from build123d import *

# Parameters (mm, degrees)
BOSS_EXTRUDE1_DEPTH          = 75
SKETCH2_R                    = 2
CUT_EXTRUDE1_DEPTH           = 15
SKETCH4_R                    = 2
CUT_EXTRUDE2_DEPTH           = 12
SKETCH3_R                    = 2.3876
CUT_EXTRUDE3_DEPTH           = 6.35
CUT_EXTRUDE3_DRAFT           = -8
CUT_EXTRUDE3_PROFILE_2_DEPTH = 6.35
CUT_EXTRUDE3_PROFILE_2_DRAFT = -8
CUT_EXTRUDE4_START           = -3
CUT_EXTRUDE4_DEPTH           = 3
CUT_EXTRUDE5_START           = -3
CUT_EXTRUDE5_DEPTH           = 3
CUT_EXTRUDE6_START           = -3
CUT_EXTRUDE6_DEPTH           = 3
CUT_EXTRUDE7_START           = -3
CUT_EXTRUDE7_DEPTH           = 3
SKETCH9_R                    = 1.4951657
CUT_EXTRUDE8_DEPTH           = 5
MIRROR2_COPY_1_SKETCH_R      = 2.3876
MIRROR2_COPY_1_DEPTH         = 6.35
MIRROR2_COPY_1_DRAFT         = -8
MIRROR2_COPY_2_SKETCH_R      = 2.3876
MIRROR2_COPY_2_DEPTH         = 6.35
MIRROR2_COPY_2_DRAFT         = -8
MIRROR2_COPY_3_SKETCH_R      = 2.3876
MIRROR2_COPY_3_DEPTH         = 6.35
MIRROR2_COPY_3_DRAFT         = -8
FILLET2_START                = 9
FILLET2_DEPTH                = 4.666666667
FILLET2_START_2              = 4
FILLET2_2_DEPTH              = 39
FILLET3_R                    = 2
SKETCH10_W                   = 1.7
SKETCH10_H                   = 63
CUT_EXTRUDE9_DEPTH           = 5
FILLET4_R                    = 1
SKETCH11_W                   = 10.2
SKETCH11_H                   = 17.7
CUT_EXTRUDE10_DEPTH          = 15
SKETCH12_R                   = 1.397
CUT_EXTRUDE11_DEPTH          = 10
FILLET5_R                    = 1
CUT_EXTRUDE12_START          = -5
CUT_EXTRUDE12_DEPTH          = 3


with BuildPart() as part:
    # Sketch1 → Boss-Extrude1 (new body)
    with BuildSketch(Plane(origin=(0, 0, 0), x_dir=(1, 0, 0), z_dir=(0, 1, 0))):
        with BuildLine():
            Line((-6.825, -6.666666667), (-6.825, -26.666666667))
            Line((-6.825, -26.666666667), (8.175, -26.666666667))
            Line((8.175, -26.666666667), (8.175, -13.175))
            Line((8.175, -13.175), (60, -13.175))
            Line((60, -13.175), (60, -1.175))
            Line((60, -1.175), (25, -1.175))
            Line((25, -1.175), (25, 2))
            ThreePointArc((25, 2), (14.923352523, 3.572976633), (5.805515239, 8.142235123))
            ThreePointArc((5.805515239, 8.142235123), (3.047757271, 9.524241472), (0, 10))
            ThreePointArc((0, 10), (-7.071067812, 7.071067812), (-10, 0))
            Line((-10, 0), (-10, -6.666666667))
            Line((-10, -6.666666667), (-6.825, -6.666666667))
        make_face()
    extrude(amount=BOSS_EXTRUDE1_DEPTH)

    # Sketch2 → Cut-Extrude1 (cut)
    with BuildSketch(Plane.ZY.offset(6.825)):
        with Locations((15.666666667, 65)):
            Circle(SKETCH2_R)
    cut_extrude1 = extrude(amount=-CUT_EXTRUDE1_DEPTH, mode=Mode.SUBTRACT)

    # Sketch4 → Cut-Extrude2 (cut)
    with BuildSketch(Plane(origin=(0, 0, 1.175), x_dir=(-1, 0, 0), z_dir=(0, 0, -1))):
        with Locations((-45, 65)):
            Circle(SKETCH4_R)
    cut_extrude2 = extrude(amount=-CUT_EXTRUDE2_DEPTH, mode=Mode.SUBTRACT)


with BuildPart() as cut_extrude3_tool:
    # Sketch3 → Cut-Extrude3 (with draft: the straight prism first)
    with BuildSketch(Plane(origin=(0, 75, 0), x_dir=(1, 0, 0), z_dir=(0, 1, 0))):
        with Locations((1, -1)):
            Circle(SKETCH3_R)
    extrude(amount=-CUT_EXTRUDE3_DEPTH)
    # Cut-Extrude3: the draft: its side faces are tilted about the plane it starts from
    cut_extrude3_sides = [cut_extrude3_tool.faces().sort_by_distance(p)[0] for p in [
        (-1.3876, 71.825, 1),
    ]]
    draft(cut_extrude3_sides, Plane(origin=(0, 75, 0), x_dir=(1, 0, 0), z_dir=(0, 1, 0)), CUT_EXTRUDE3_DRAFT)


with BuildPart() as part_1:
    add(part.part)

    # Cut-Extrude3: cut by cut_extrude3_tool
    add(cut_extrude3_tool.part, mode=Mode.SUBTRACT)


with BuildPart() as cut_extrude3_profile_2_tool:
    # Sketch3 → Cut-Extrude3 profile 2 (with draft: the straight prism first)
    with BuildSketch(Plane(origin=(0, 75, 0), x_dir=(1, 0, 0), z_dir=(0, 1, 0))):
        with Locations((30, -7.175)):
            Circle(SKETCH3_R)
    extrude(amount=-CUT_EXTRUDE3_PROFILE_2_DEPTH)
    # Cut-Extrude3 profile 2: the draft: its side faces are tilted about the plane it starts from
    cut_extrude3_profile_2_sides = [cut_extrude3_profile_2_tool.faces().sort_by_distance(p)[0] for p in [
        (27.6124, 71.825, 7.175),
    ]]
    draft(cut_extrude3_profile_2_sides, Plane(origin=(0, 75, 0), x_dir=(1, 0, 0), z_dir=(0, 1, 0)), CUT_EXTRUDE3_PROFILE_2_DRAFT)


with BuildPart() as part_2:
    add(part_1.part)

    # Cut-Extrude3 profile 2: cut by cut_extrude3_profile_2_tool
    add(cut_extrude3_profile_2_tool.part, mode=Mode.SUBTRACT)

    # Sketch5 → Cut-Extrude4 (cut)
    with BuildSketch(Plane(origin=(8.175, 0, 0), x_dir=(0, 0, -1), z_dir=(1, 0, 0)).offset(CUT_EXTRUDE4_START)):
        Polygon((-19.885416667, 62.564303552), (-15.666666667, 60.128607104), (-11.447916667, 62.564303552), (-11.447916667, 75), (-19.885416667, 75), align=None)
    cut_extrude4 = extrude(amount=-CUT_EXTRUDE4_DEPTH, mode=Mode.SUBTRACT)

    # Sketch6 → Cut-Extrude5 (cut)
    with BuildSketch(Plane(origin=(8.175, 0, 0), x_dir=(0, 0, -1), z_dir=(1, 0, 0)).offset(CUT_EXTRUDE5_START)):
        with BuildLine():
            Line((-13.666666667, 65), (-13.666666667, 75))
            Line((-13.666666667, 75), (-17.666666667, 75))
            Line((-17.666666667, 75), (-17.666666667, 65))
            ThreePointArc((-17.666666667, 65), (-15.666666667, 67), (-13.666666667, 65))
        make_face()
    cut_extrude5 = extrude(amount=CUT_EXTRUDE5_DEPTH, mode=Mode.SUBTRACT)

    # Sketch7 → Cut-Extrude6 (cut)
    with BuildSketch(Plane.XY.offset(13.175).offset(CUT_EXTRUDE6_START)):
        Polygon((40.78125, 62.564303552), (45, 60.128607104), (49.21875, 62.564303552), (49.21875, 75), (40.78125, 75), align=None)
    cut_extrude6 = extrude(amount=-CUT_EXTRUDE6_DEPTH, mode=Mode.SUBTRACT)

    # Sketch8 → Cut-Extrude7 (cut)
    with BuildSketch(Plane.XY.offset(13.175).offset(CUT_EXTRUDE7_START)):
        with BuildLine():
            Line((47, 65), (47, 75))
            Line((47, 75), (43, 75))
            Line((43, 75), (43, 65))
            ThreePointArc((43, 65), (45, 67), (47, 65))
        make_face()
    cut_extrude7 = extrude(amount=CUT_EXTRUDE7_DEPTH, mode=Mode.SUBTRACT)

    # Sketch9 → Cut-Extrude8 (cut)
    with BuildSketch(Plane(origin=(0, 68.65, 0), x_dir=(1, 0, 0), z_dir=(0, 1, 0))):
        with Locations(Location((1, -1, 0), (0, 0, 270))):
            Circle(SKETCH9_R)
        with Locations(Location((30, -7.175, 0), (0, 0, 270))):
            Circle(SKETCH9_R)
    cut_extrude8 = extrude(amount=-CUT_EXTRUDE8_DEPTH, mode=Mode.SUBTRACT)

    # Mirror2: Cut-Extrude1, Cut-Extrude2, Cut-Extrude4, Cut-Extrude5, Cut-Extrude6, Cut-Extrude7, Cut-Extrude8 across plane
    add(cut_extrude1.mirror(Plane.ZX.offset(37.5)), mode=Mode.SUBTRACT)
    add(cut_extrude2.mirror(Plane.ZX.offset(37.5)), mode=Mode.SUBTRACT)
    add(cut_extrude4.mirror(Plane.ZX.offset(37.5)), mode=Mode.SUBTRACT)
    add(cut_extrude5.mirror(Plane.ZX.offset(37.5)), mode=Mode.SUBTRACT)
    add(cut_extrude6.mirror(Plane.ZX.offset(37.5)), mode=Mode.SUBTRACT)
    add(cut_extrude7.mirror(Plane.ZX.offset(37.5)), mode=Mode.SUBTRACT)
    add(cut_extrude8.mirror(Plane.ZX.offset(37.5)), mode=Mode.SUBTRACT)


with BuildPart() as mirror2_copy_1_tool:
    # Mirror2 copy 1 sketch → Mirror2 copy 1 (with draft: the straight prism first)
    with BuildSketch(Plane.XZ):
        with Locations((1, 1)):
            Circle(MIRROR2_COPY_1_SKETCH_R)
    extrude(amount=-MIRROR2_COPY_1_DEPTH)
    # Mirror2 copy 1: the draft: its side faces are tilted about the plane it starts from
    mirror2_copy_1_sides = [mirror2_copy_1_tool.faces().sort_by_distance(p)[0] for p in [
        (-1.3876, 3.175, 1),
    ]]
    draft(mirror2_copy_1_sides, Plane.XZ, MIRROR2_COPY_1_DRAFT)


with BuildPart() as part_3:
    add(part_2.part)

    # Mirror2 copy 1: cut by mirror2_copy_1_tool
    add(mirror2_copy_1_tool.part, mode=Mode.SUBTRACT)


with BuildPart() as mirror2_copy_2_tool:
    # Mirror2 copy 2 sketch → Mirror2 copy 2 (with draft: the straight prism first)
    with BuildSketch(Plane.XZ):
        with Locations((30, 7.175)):
            Circle(MIRROR2_COPY_2_SKETCH_R)
    extrude(amount=-MIRROR2_COPY_2_DEPTH)
    # Mirror2 copy 2: the draft: its side faces are tilted about the plane it starts from
    mirror2_copy_2_sides = [mirror2_copy_2_tool.faces().sort_by_distance(p)[0] for p in [
        (27.6124, 3.175, 7.175),
    ]]
    draft(mirror2_copy_2_sides, Plane.XZ, MIRROR2_COPY_2_DRAFT)


with BuildPart() as part_4:
    add(part_3.part)

    # Mirror2 copy 2: cut by mirror2_copy_2_tool
    add(mirror2_copy_2_tool.part, mode=Mode.SUBTRACT)


with BuildPart() as mirror2_copy_3_tool:
    # Mirror2 copy 3 sketch → Mirror2 copy 3 (with draft: the straight prism first)
    with BuildSketch(Plane.XZ):
        with Locations((30, 7.175)):
            Circle(MIRROR2_COPY_3_SKETCH_R)
    extrude(amount=-MIRROR2_COPY_3_DEPTH)
    # Mirror2 copy 3: the draft: its side faces are tilted about the plane it starts from
    mirror2_copy_3_sides = [mirror2_copy_3_tool.faces().sort_by_distance(p)[0] for p in [
        (27.6124, 3.175, 7.175),
    ]]
    draft(mirror2_copy_3_sides, Plane.XZ, MIRROR2_COPY_3_DRAFT)


with BuildPart() as part_5:
    add(part_4.part)

    # Mirror2 copy 3: cut by mirror2_copy_3_tool
    add(mirror2_copy_3_tool.part, mode=Mode.SUBTRACT)

    # Fillet2: read off the stored shape, not the designer's step
    # Fillet2 outline → Fillet2 (cut)
    with BuildSketch(Plane.XY.offset(FILLET2_START)):
        with BuildLine():
            Line((47, 1), (47, 0))
            Line((47, 0), (48, 0))
            ThreePointArc((48, 0), (47.292893219, 0.292893219), (47, 1))
        make_face()
        with BuildLine():
            Line((48, 75), (47, 75))
            Line((47, 75), (47, 74))
            ThreePointArc((47, 74), (47.292893219, 74.707106781), (48, 75))
        make_face()
        with BuildLine():
            Line((43, 75), (42, 75))
            ThreePointArc((42, 75), (42.707106781, 74.707106781), (43, 74))
            Line((43, 74), (43, 75))
        make_face()
        with BuildLine():
            ThreePointArc((43, 1), (42.707106781, 0.292893219), (42, 0))
            Line((42, 0), (43, 0))
            Line((43, 0), (43, 1))
        make_face()
    extrude(amount=FILLET2_DEPTH, mode=Mode.SUBTRACT)

    # Fillet2 2 outline → Fillet2 2 (cut)
    with BuildSketch(Plane.YZ.offset(FILLET2_START_2)):
        with BuildLine():
            Line((74, 17.666666667), (75, 17.666666667))
            Line((75, 17.666666667), (75, 18.666666667))
            ThreePointArc((75, 18.666666667), (74.707106782, 17.959559886), (74, 17.666666667))
        make_face()
        with BuildLine():
            ThreePointArc((74, 13.666666667), (74.707106781, 13.373773448), (75, 12.666666667))
            Line((75, 12.666666667), (75, 13.666666667))
            Line((75, 13.666666667), (74, 13.666666667))
        make_face()
        with BuildLine():
            ThreePointArc((1, 17.666666667), (0.292893218, 17.959559886), (0, 18.666666667))
            Line((0, 18.666666667), (0, 17.666666667))
            Line((0, 17.666666667), (1, 17.666666667))
        make_face()
    extrude(amount=FILLET2_2_DEPTH, mode=Mode.SUBTRACT)

    # Fillet3
    fillet3_edges = [part_5.edges().sort_by_distance(p)[0] for p in [
        (60, 0, 7.175),
        (0.675, 0, 26.666666667),
        (60, 37.5, 1.175),
        (60, 37.5, 13.175),
        (8.175, 37.5, 26.666666667),
        (-6.825, 37.5, 26.666666667),
        (0.675, 75, 26.666666667),
        (60, 75, 7.175),
    ]]
    fillet(fillet3_edges, radius=FILLET3_R)

    # Sketch10 → Cut-Extrude9 (cut)
    with BuildSketch(Plane(origin=(60, 0, 0), x_dir=(0, 0, -1), z_dir=(1, 0, 0))):
        with Locations((-6.175, 31.5)):
            Rectangle(SKETCH10_W, SKETCH10_H)
    extrude(amount=-CUT_EXTRUDE9_DEPTH, mode=Mode.SUBTRACT)

    # Fillet4
    fillet4_edges = [part_5.edges().sort_by_distance(p)[0] for p in [
        (59.414213562, 0.585786438, 7.025),
        (59.414213562, 0.585786438, 5.325),
        (60, 32.5, 7.025),
        (60, 32.5, 5.325),
        (55, 0, 6.175),
        (56.5, 0, 5.325),
        (56.5, 0, 7.025),
    ]]
    fillet(fillet4_edges, radius=FILLET4_R)

    # Sketch11 → Cut-Extrude10 (cut)
    with BuildSketch(Plane(origin=(8.175, 0, 0), x_dir=(0, 0, -1), z_dir=(1, 0, 0))):
        with Locations((-18.275, 36.85)):
            Rectangle(SKETCH11_W, SKETCH11_H)
    extrude(amount=-CUT_EXTRUDE10_DEPTH, mode=Mode.SUBTRACT)

    # Sketch12 → Cut-Extrude11 (cut)
    with BuildSketch(Plane.XY.offset(13.175)):
        with Locations((18.175, 17)):
            Circle(SKETCH12_R)
        with Locations((18.175, 56.7)):
            Circle(SKETCH12_R)
    extrude(amount=-CUT_EXTRUDE11_DEPTH, mode=Mode.SUBTRACT)

    # Fillet5
    fillet5_edges = [part_5.edges().sort_by_distance(p)[0] for p in [
        (0.675, 45.7, 13.175),
        (0.675, 28, 13.175),
        (0.675, 28, 23.375),
        (0.675, 45.7, 23.375),
    ]]
    fillet(fillet5_edges, radius=FILLET5_R)

    # Sketch13 → Cut-Extrude12 (cut)
    with BuildSketch(Plane.XZ.offset(CUT_EXTRUDE12_START)):
        Polygon((-2.893869279, -1.927157459), (1.588058081, -3.835768444), (5.48192736, -0.908610985), (24.216737808, 13.175), (10.175, 13.175), (0.411941919, 5.835768444), (-3.48192736, 2.908610985), align=None)
    extrude(amount=-CUT_EXTRUDE12_DEPTH, mode=Mode.SUBTRACT)


solid = part_5.part
Geometry: final body of the model. Coordinates: model frame, mm. A direction names the side the tool comes from. Round coordinates to 2 decimals unless told otherwise and drop trailing zeros. Order: outer loops, then holes, each group sorted by start corner. A loop starts at its lowest first (then second) coordinate and runs counter-clockwise, first axis right, second up.
Q1. Access query for faces 4 (the face through (1, 28, 18)), 5 (the face through (7, 8, 7)), 6 (the face through (30, 63.65, 7)). Directions: +Z, -Z, +X, -X, +Y, -Y. A direction counts if a zero-diameter tool reaches every point of the face in a straight line with its end or side. Return the directions, or none.
Result sheet:
face 4: +X, -X
face 5: none
face 6: +Y
Q2. Section C-C, the plane x = 12.5. Output: boundary loops of the cut face in (y, z) (3 decimals), and give its area (3 significant figures).
Result sheet:
outline: (0, -4.454) - (75, -4.454) - (75, 12.667) arc R1 ccw to (74.861, 13.175) - (8, 13.175) - (8, 4.367) - (5, 4.367) - (5, 13.175) - (0, 13.175) - close
area: 1,300 mm2
Q3. Section B-B, the plane y = 56.7. Output: boundary loops of the cut face in (x, z) (1 decimal), and give its area (3 significant figures).
Result sheet:
outline: (-10, 0) arc R10 ccw to (5.8, -8.1) arc R33.1 cw to (25, -2) - (25, 1.2) - (58, 1.2) arc R2 ccw to (60, 3.2) - (60, 4.3) arc R1 ccw to (59, 5.3) - (55, 5.3) - (55, 7) - (59, 7) arc R1 ccw to (60, 8) - (60, 11.2) arc R2 ccw to (58, 13.2) - (19.6, 13.2) - (19.6, 3.2) - (16.8, 3.2) - (16.8, 13.2) - (8.2, 13.2) - (8.2, 24.7) arc R2 ccw to (6.2, 26.7) - (-4.8, 26.7) arc R2 ccw to (-6.8, 24.7) - (-6.8, 6.7) - (-10, 6.7) - close
area: 1,230 mm2
Q4. Material intervals for probe 1 along Z at (x, y) = (30, 9.4) (3 decimals); probe 2 along Z at (x, y) = (57, 5) (3 decimals); probe 3 along Z at (x, y) = (1, 9.5), sorted ascending.
Result sheet:
probe 1: z = 1.175 to 5.68, 8.67 to 13.175
probe 2: z = 1.175 to 5.325, 7.025 to 13.175
probe 3: z = -9.95 to -0.5, 2.5 to 13.73, 17.6 to 26.67
Q5. Pin query (flat end, axial travel): pin 1 (7 mm diameter, centred on x = 46, y = 7.5, fed in from -Z) (3 decimals); pin 2 (2 mm diameter, centred on y = 34.5, z = 10.5, fed in from -X) (3 decimals); pin 3 (3.5 mm diameter, centred on x = 3, y = 3.5, fed in from -Z); pin 4 (2.5 mm diameter, centred on y = 69, z = 11.5, fed in from +X). Return the tip coordinate at first contact, or that it passes through.
Result sheet:
pin 1: stops at z = 1.175
pin 2: stops at x = -6.825
pin 3: stops at z = -9.92
pin 4: stops at x = 60
Q6. Section D-D, the plane y = 25. Output: boundary loops of the cut face in (x, z) (1 decimal).
Result sheet:
outline: (-10, 0) arc R10 ccw to (5.8, -8.1) arc R33.1 cw to (25, -2) - (25, 1.2) - (58, 1.2) arc R2 ccw to (60, 3.2) - (60, 4.3) arc R1 ccw to (59, 5.3) - (55, 5.3) - (55, 7) - (59, 7) arc R1 ccw to (60, 8) - (60, 11.2) arc R2 ccw to (58, 13.2) - (8.2, 13.2) - (8.2, 24.7) arc R2 ccw to (6.2, 26.7) - (-4.8, 26.7) arc R2 ccw to (-6.8, 24.7) - (-6.8, 6.7) - (-10, 6.7) - close
Q7. Mould query, pull axis Y, two halves, no side actions, for faces 1 (the face through (-0.68, 6.48, -2.87)), 2 (the face through (47.08, 61.33, 8.7)), 3 (the face through (2.175, 6, 16)). Classes: released by +Y, released by -Y, zero draft, split by the parting line, or undercut.
Result sheet:
face 1: undercut
face 2: released by +Y
face 3: zero draft
Q8. Section A-A, the plane y = 36. Output: boundary loops of the cut face in (x, z) (1 decimal).
Result sheet:
outline: (-10, 0) arc R10 ccw to (5.8, -8.1) arc R33.1 cw to (25, -2) - (25, 1.2) - (58, 1.2) arc R2 ccw to (60, 3.2) - (60, 4.3) arc R1 ccw to (59, 5.3) - (55, 5.3) - (55, 7) - (59, 7) arc R1 ccw to (60, 8) - (60, 11.2) arc R2 ccw to (58, 13.2) - (-6.8, 13.2) - (-6.8, 6.7) - (-10, 6.7) - close; (-6.8, 23.4) - (8.2, 23.4) - (8.2, 24.7) arc R2 ccw to (6.2, 26.7) - (-4.8, 26.7) arc R2 ccw to (-6.8, 24.7) - close
